Could you check a few things on this model? Use its own coordinates, in mm. A direction names the side the tool comes from. Round coordinates to 2 decimals unless told otherwise and drop trailing zeros. Loops run counter-clockwise (first coordinate to the right, second up) from the corner with the lowest first, then second, coordinate; pieces in that order, holes last. Notation, with made-up numbers: (-24.75, 31.5) - (28.25, 31.5) arc R16 ccw to (28.25, 45.5) - close; hole circle Ø3 at (-37.5, 16.25). An arc over 180 degrees is marked (long way). Answer as CSV lines item,"result". Start each with the question number.
1) Which directions (+Z, -Z, +X, -X, +Y, -Y) give clear straight access to the entire face, cutting with the end or side of a thin tool? Please do faces 1 (the face through (116, 77.718, 1)), 2 (the face through (179, 77.718, 1)), 3 (the face through (160, 74, 3)), 4 (the face through (117, 69.718, 1)).
2) Suppose I cut it at C-C, the plane x = 169.5. Write out the boundary of the cut face in (y, z).
3) We'd pull the mould along Y, two halves only. Please class faces 5 (the face through (102.602, 72.387, 1.479)), 6 (the face through (141.583, 77.897, 1.479)), 7 (the face through (97.91, 73.63, 1.48)), 8 (the face through (180, 69.718, 1)): pulls with the +Y half, pulls with the -Y half, needs draft (parallel to the pull), parting line crosses it, or undercut.
4) Suppose I cut it at A-A, the plane x = 137. Write out the boundary of the cut face in (y, z).
5) I'm going to push flat-ended pins straight in: pin 1 Ø0.9 at (x, z) = (176.5, 1.5) entering from +Y; pin 2 Ø2.5 at (x, y) = (136.91, 73.75) entering from +Z; pin 3 Ø0.9 at (x, z) = (115, 1) entering from -Y; pin 4 Ø1.5 at (y, z) = (71, 2) entering from +X. Where does each tip first touch, or does it pass through?
6) Suppose I cut it at B-B, the plane z = 1.8. Write out the boundary of the cut face in (x, y), then the cut area to 3 significant figures.
7) Please list where these lines run through material, in increasing order: line 1 along Y through (x, z) = (137, 0.3); line 2 along X through (y, z) = (72.75, 1.95); line 3 along Y through (x, z) = (214.5, 1).
```python
from build123d import *

# Parameters (mm, degrees)
ESQUISSE15_R        = 1.5
BOSS_EXTRU_15_DEPTH = 3


with BuildPart() as part:
    # Esquisse15 → Boss.-Extru.15 (new body)
    with BuildSketch(Plane.XY):
        with BuildLine():
            Line((101.910180697, 77.71752531), (131.216827386, 77.71752531))
            ThreePointArc((131.216827386, 77.71752531), (132.224213524, 77.891720439), (133.114611823, 78.394076531))
            ThreePointArc((133.114611823, 78.394076531), (136.910180697, 79.747178972), (140.705749571, 78.394076531))
            ThreePointArc((140.705749571, 78.394076531), (141.59614787, 77.891720439), (142.603534008, 77.71752531))
            Line((142.603534008, 77.71752531), (216.910180697, 77.71752531))
            ThreePointArc((216.910180697, 77.71752531), (220.910180697, 73.71752531), (216.910180697, 69.71752531))
            Line((216.910180697, 69.71752531), (142.530142387, 69.71752531))
            ThreePointArc((142.530142387, 69.71752531), (141.537583488, 69.54857226), (140.656821824, 69.060743198))
            ThreePointArc((140.656821824, 69.060743198), (136.910180697, 67.747178972), (133.16353957, 69.060743198))
            ThreePointArc((133.16353957, 69.060743198), (132.282777907, 69.54857226), (131.290219007, 69.71752531))
            Line((131.290219007, 69.71752531), (101.910180697, 69.71752531))
            ThreePointArc((101.910180697, 69.71752531), (97.910180697, 73.71752531), (101.910180697, 77.71752531))
        make_face()
        with Locations((101.910180697, 73.71752531)):
            Circle(ESQUISSE15_R, mode=Mode.SUBTRACT)
        with Locations((216.910180697, 73.71752531)):
            Circle(ESQUISSE15_R, mode=Mode.SUBTRACT)
        with Locations((136.910180697, 73.747178972)):
            Circle(ESQUISSE15_R, mode=Mode.SUBTRACT)
    extrude(amount=BOSS_EXTRU_15_DEPTH)


solid = part.part
```
Filled sheet:
1,face 1,"+Z, -Z, -X, +Y"
1,face 2,"+Z, -Z, +X, +Y"
1,face 3,"+Z, +X, -X, +Y, -Y"
1,face 4,"+Z, -Z, -X, -Y"
2,outline,"(69.72, 0) - (77.72, 0) - (77.72, 3) - (69.72, 3) - close"
3,face 5,"undercut"
3,face 6,"pulls with the +Y half"
3,face 7,"parting line crosses it"
3,face 8,"pulls with the -Y half"
4,outline,"(67.75, 0) - (72.25, 0) - (72.25, 3) - (67.75, 3) - close; (75.24, 0) - (79.75, 0) - (79.75, 3) - (75.24, 3) - close"
5,pin 1,"y = 77.72"
5,pin 2,"through"
5,pin 3,"y = 69.72"
5,pin 4,"x = 220.39"
6,outline,"(101.91, 69.72) - (131.29, 69.72) arc R3 cw to (133.16, 69.06) arc R6 ccw to (140.66, 69.06) arc R3 cw to (142.53, 69.72) - (216.91, 69.72) arc R4 ccw to (216.91, 77.72) - (142.6, 77.72) arc R3 cw to (140.71, 78.39) arc R6 ccw to (133.11, 78.39) arc R3 cw to (131.22, 77.72) - (101.91, 77.72) arc R4 ccw to start; hole circle Ø3 at (101.91, 73.72); hole circle Ø3 at (136.91, 73.75); hole circle Ø3 at (216.91, 73.72)"
6,area,"974 mm²"
7,line 1,"67.75 to 72.25, 75.24 to 79.75"
7,line 2,"98.03 to 100.76, 103.06 to 135.79, 138.03 to 215.76, 218.06 to 220.79"
7,line 3,"69.72 to 77.72"
